Build history of the part. All positions in model axes, mm. A direction names the side the tool comes from. Give positions to 0.01 mm unless a question says otherwise; leave off trailing zeros. Loops run counter-clockwise (first coordinate to the right, second up) from the corner with the lowest first, then second, coordinate; pieces in that order, holes last. Notation, with made-up numbers: (20, 0) - (39, 0) arc R8 ccw to (39, 9) - close; hole circle Ø1 at (-27, -31.75). An arc over 180 degrees is marked (long way). Return JSON: item names as keys, results as strings. Group by question number.
1) Drop flat-ended pins along their axis: pin 1 (3 mm diameter, centred on x = 0.5, z = 388.5, fed in from +Y); pin 2 (1.1 mm diameter, centred on x = 0.5, y = 9.5, fed in from +Z); pin 3 (1.1 mm diameter, centred on x = 1, y = -9, fed in from +Z). Give the stop position or say it passes through.
2) Mould opens along Z. For faces 5 (the face through (0, 0, 100)), 6 (the face through (7.535, 4.27, 385.14)), 7 (the face through (-2.17, -9.76, 421.87)) say: released by +Z, released by -Z, zero draft, split by the parting line, or undercut.
3) 3-axis set-ups, long thin cutter, end or side, ignore diameter. For faces 1 (the face through (0, -8.66, 385)), 2 (the face through (-7.535, -4.27, 385.14)), 3 (the face through (0, 8.66, 385)), 4 (the face through (-7.465, 4.391, 385.14)): which of +Z, -Z, +X, -X, +Y, -Y reach the whole face in a straight line?
4) Drill centre lines: probe 1 along Y at (x, z) = (-1, 287); probe 2 along Y at (x, z) = (-4.25, 384.5); probe 3 along X at (y, z) = (-8.75, 195.5). Where is each one in solid material? Low to high. Write a range as from..to.
5) Slice it at B-B (z = 462). List the corners of the cut face in (x, y).
```python
from build123d import *

# Parameters (mm, degrees)
SKETCH1_R          = 10
EXTRUDE1_DEPTH     = 500
CHAMFER1_SIZE      = 2
SKETCH2_R          = 43.013092774
SKETCH2_R_2        = 8
CUT_EXTRUDE1_DEPTH = 50
CHAMFER2_SIZE      = 2
SKETCH3_R          = 224.622331413
REMOVE_DEPTH       = 600
SKETCH4_R          = 20
HEX_2_DEPTH        = 20
CHAMFER3_SIZE      = 5
CHAMFER3_SIZE2     = 57.150261514


with BuildPart() as part:
    # Sketch1 → Extrude1 (new, symmetric)
    with BuildSketch(Plane.XY):
        Circle(SKETCH1_R)
    extrude(amount=EXTRUDE1_DEPTH, both=True)

    # Chamfer1
    chamfer1_edges = [part.edges().sort_by_distance(p)[0] for p in [
        (-10, 0, -500),
        (-10, 0, 500),
    ]]
    chamfer(chamfer1_edges, length=CHAMFER1_SIZE)

    # Sketch2 → Cut-Extrude1 (cut)
    with BuildSketch(Plane.XY.offset(500)):
        Circle(SKETCH2_R)
        Circle(SKETCH2_R_2, mode=Mode.SUBTRACT)
    extrude(amount=-CUT_EXTRUDE1_DEPTH, mode=Mode.SUBTRACT)

    # Chamfer2
    chamfer2_edges = [part.edges().sort_by_distance(p)[0] for p in [
        (-10, 0, 450),
    ]]
    chamfer(chamfer2_edges, length=CHAMFER2_SIZE - 0.0001)  # a hair under: the kernel refuses the full size

    # Sketch3 → remove (cut)
    with BuildSketch(Plane(origin=(0, 0, -500), x_dir=(-1, 0, 0), z_dir=(0, 0, -1))):
        Circle(SKETCH3_R)
    extrude(amount=-REMOVE_DEPTH, mode=Mode.SUBTRACT)

    # Sketch4 → hex 2 (cut)
    with BuildSketch(Plane.XY.offset(395)):
        Circle(SKETCH4_R)
        Polygon((5, 8.660254038), (-5, 8.660254038), (-10, 0), (-5, -8.660254038), (5, -8.660254038), (10, 0), align=None, mode=Mode.SUBTRACT)
    extrude(amount=-HEX_2_DEPTH, mode=Mode.SUBTRACT)

    # Chamfer3
    chamfer3_edges = [part.edges().sort_by_distance(p)[0] for p in [
        (-10, 0, 100),
    ]]
    chamfer3_side = [part.faces().sort_by_distance(p)[0] for p in [
        (0, 0, 100),
    ]]
    chamfer(chamfer3_edges, length=CHAMFER3_SIZE, length2=CHAMFER3_SIZE2, reference=chamfer3_side[0])


solid = part.part
```
Results:
{
 "1": {"pin 1": "y = 8.66", "pin 2": "z = 449.04", "pin 3": "z = 449.49"},
 "2": {"face 5": "released by -Z", "face 6": "undercut", "face 7": "zero draft"},
 "3": {"face 1": "+X, -X, -Y", "face 2": "-X, -Y", "face 3": "+X, -X, +Y", "face 4": "-X, +Y"},
 "4": {"probe 1": "-9.95..9.95", "probe 2": "-8.66..8.66", "probe 3": "-4.84..4.84"},
 "5": {"outline": "circle Ø16 at (0, 0)"}
}
